from build123d import *

# Parameters (mm, degrees)
PAD_DEPTH         = 1
SKETCH001_W       = 3
SKETCH001_H       = 1
SKETCH001_W_2     = 3.012331
SKETCH001_W_3     = 2.553459
SKETCH001_H_2     = 1.5
PAD001_DEPTH      = 20
CYLINDER_R        = 3.05
CYLINDER_DEPTH    = 15
CYLINDER002_R     = 3.05
CYLINDER002_DEPTH = 15
PAD002_DEPTH      = 5
CYLINDER001_R     = 3.05
CYLINDER001_DEPTH = 15


with BuildPart() as channels_with_connection:
    # Sketch → Pad (new body)
    with BuildSketch(Plane.XY.offset(2)):
        Polygon((-1.5, 0), (1.5, 0), (1.5, -100), (-1.5, -100), (-1.5, -26.5), (-21.5, -26.5), (-21.5, -25), (-1.5, -25), align=None)
    extrude(amount=PAD_DEPTH)

    # Sketch001 → Pad001 (new body)
    with BuildSketch(Plane.XY.offset(3)):
        with Locations((0, -0.5)):
            Rectangle(SKETCH001_W, SKETCH001_H)
        with Locations((0.001527, -99.493348)):
            Rectangle(SKETCH001_W_2, SKETCH001_H)
        with Locations((-20.22327, -25.757023)):
            Rectangle(SKETCH001_W_3, SKETCH001_H_2)
    extrude(amount=PAD001_DEPTH)


with BuildPart() as cylinder:
    # Cylinder → Cylinder (new body)
    with BuildSketch(Plane(origin=(0, -0.5, 0), x_dir=(1, 0, 0), z_dir=(0, 0, 1))):
        Circle(CYLINDER_R)
    extrude(amount=CYLINDER_DEPTH)


with BuildPart() as cylinder002:
    # Cylinder002 → Cylinder002 (new body)
    with BuildSketch(Plane(origin=(-20.4, -25.6, 0), x_dir=(1, 0, 0), z_dir=(0, 0, 1))):
        Circle(CYLINDER002_R)
    extrude(amount=CYLINDER002_DEPTH)


with BuildPart() as volume_medium:
    # Sketch002 → Pad002 (new body)
    with BuildSketch(Plane.XY):
        Polygon((-6.5, 5), (6.5, 5), (6.5, -105), (-6.5, -105), (-6.5, -32.25), (-25, -32.25), (-25, -19.25), (-6.5, -19.25), align=None)
    extrude(amount=PAD002_DEPTH)


with BuildPart() as t_junction:
    # Cylinder001 → Cylinder001 (new body)
    with BuildSketch(Plane(origin=(0, -99.5, 0), x_dir=(1, 0, 0), z_dir=(0, 0, 1))):
        Circle(CYLINDER001_R)
    extrude(amount=CYLINDER001_DEPTH)

    # Fusion: union Cylinder, Cylinder002, volume_medium
    add(cylinder.part)
    add(cylinder002.part)
    add(volume_medium.part)

    # Cut: cut channels_with_connection
    add(channels_with_connection.part, mode=Mode.SUBTRACT)


solid = t_junction.part
Geometry check sheet. Reference: the model listing, model coordinates, mm. A direction names the side the tool comes from. Coordinates: 2 decimals unless noted, no trailing zeros. Order: outer loops, then holes, each group sorted by start corner. A loop starts at its lowest first (then second) coordinate and runs counter-clockwise, first axis right, second up. Notation, with made-up numbers: (-34, 81) -> (6, 81) arc R14 cw to (6, 97) -> close; hole circle Ø8 at (1, 88). An arc over 180 degrees is marked (long way). Use a Markdown table: item, result. Add a question column.
1. Cross-section at A-A (z = 13.5). Enter the section's corners in (x, y), and give its area (3 significant figures).
2. Cross-section at C-C (y = -82). Enter the section's corners in (x, z), and give its area (3 significant figures).
3. Mould release check, pull along Z, two halves, no side actions. Record for faces 1 (the face through (0, -50, 2)), 2 (the face through (0, -98.993, 9)), 3 (the face through (-2, -49, 5)): pulls with the +Z half, pulls with the -Z half, needs draft (parallel to the pull), parting line crosses it, or undercut.
4. Material ranges on L1, parallel to Y at x = 1, z = 4.75; L2, parallel to Y at x = -2, z = 2.25; L3, parallel to Y at x = 0, z = 7, recorded low to high.
5. Go/stop test with flat-tipped pins: pin 1 Ø1.6 at (y, z) = (-26, 10) entering from +X; pin 2 Ø16 at (x, y) = (-16.5, -57) entering from +Z; pin 3 Ø1.5 at (x, z) = (-20, 3.5) entering from -Y; pin 4 Ø2.5 at (x, z) = (-0.5, 11) entering from -Y. Record where each tip stops, or that it passes through.
6. Set-up check for faces 4 (the face through (-16, -32.25, 2)), 5 (the face through (1.5, -50.2, 2.7)), 6 (the face through (-16, -19.25, 2)), 7 (the face through (-18.993, -28.306, 9.93)): record each of +Z, -Z, +X, -X, +Y, -Y from which the full face is reachable in a straight line by a thin tool's end or side.
Filled sheet:
| question | item | result |
|---|---|---|
| 1 | outline | circle Ø6.1 at (-20.4, -25.6); circle Ø6.1 at (0, -99.5); circle Ø6.1 at (0, -0.5); hole (-21.5, -26.51) -> (-18.95, -26.51) -> (-18.95, -25.01) -> (-21.5, -25.01) -> close; hole (-1.5, -99.99) -> (1.51, -99.99) -> (1.51, -98.99) -> (-1.5, -98.99) -> close; hole (-1.5, -1) -> (1.5, -1) -> (1.5, 0) -> (-1.5, 0) -> close |
| 1 | area | 77.8 mm2 |
| 2 | outline | (-6.5, 0) -> (6.5, 0) -> (6.5, 5) -> (-6.5, 5) -> close; hole (-1.5, 2) -> (1.5, 2) -> (1.5, 3) -> (-1.5, 3) -> close |
| 2 | area | 62.0 mm2 |
| 3 | face 1 | undercut |
| 3 | face 2 | needs draft |
| 3 | face 3 | pulls with the +Z half |
| 4 | L1 | -105 to -99.99, -98.99 to -1, 0 to 5 |
| 4 | L2 | -105 to -26.5, -25 to 5 |
| 4 | L3 | -102.55 to -99.99, -98.99 to -96.45, -3.55 to -1, 0 to 2.55 |
| 5 | pin 1 | x = -17.35 |
| 5 | pin 2 | through |
| 5 | pin 3 | y = -32.25 |
| 5 | pin 4 | y = -102.55 |
| 6 | face 4 | +Z, -Z, -X, -Y |
| 6 | face 5 | none |
| 6 | face 6 | +Z, -Z, -X, +Y |
| 6 | face 7 | +Z |
